Check sheet for the drawn part. Datum: minimum x, y, z corner. Units: mm. A direction names the side the tool comes from. Round coordinates to 2 decimals unless told otherwise and drop trailing zeros. Answer as a JSON object with one key per item and string values. Group by question number.
1) Go/stop test with flat-tipped pins: pin 1 Ø12.5 at (x, y) = (14, 68) entering from -Z (3 decimals); pin 2 Ø12 at (x, z) = (22.5, 12.5) entering from +Y (3 decimals). Record where each tip stops, or that it passes through.
2) Mould release check, pull along X, two halves, no side actions. Record for the marked faces 3, 4 and 5: +X half, -X half, draft (parallel to the pull), parting line (faces both ways), or undercut.
3) Section check A-A (y = 146.05). State how many separate pieces and enclosed holes the cut face has, then the cut area to 3 significant figures.
4) Set-up check for the marked faces 1 and 2: record each of +Z, -Z, +X, -X, +Y, -Y from which the full face is reachable in a straight line by a thin tool's end or side.
5) Thickness scan on line 1 (Z direction, x = 2, y = 146). Record the ranges inside material, lowest first.
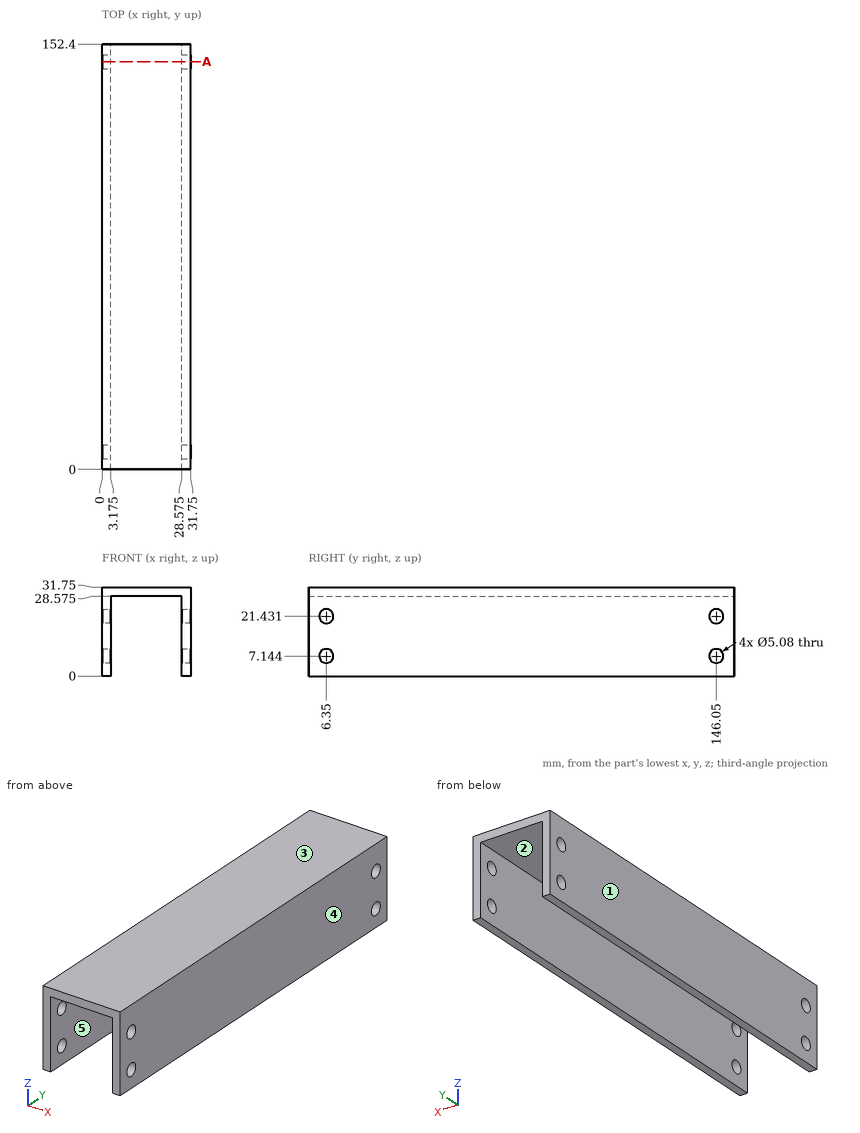
Returned:
{
 "1": {"pin 1": "z = 28.575", "pin 2": "through"},
 "2": {"face 3": "draft", "face 4": "+X half", "face 5": "undercut"},
 "3": {"separate pieces": "5", "enclosed holes": "0", "area": "218 mm2"},
 "4": {"face 1": "+Z, -Z, -X, +Y, -Y", "face 2": "-Z, +Y, -Y"},
 "5": {"line 1": "0 to 4.6, 9.68 to 18.89, 23.97 to 31.75"}
}
